Autodesk Inventor part; units mm, degrees
ref_plane "YZ Plane" through (0, 0, 0) normal (1, 0, 0) x (0, 1, 0)
ref_plane "XZ Plane" through (0, 0, 0) normal (0, 1, 0) x (-1, 0, 0)
ref_plane "XY Plane" through (0, 0, 0) normal (0, 0, 1) x (1, 0, 0)
sketch "Sketch1" plane through (0, 0, 0) normal (0, 0, 1) x (1, 0, 0)
  line L0 (0, 0) -> (30.25, 0) construction
  line L1 (0, 0) -> (-30.25, 0) construction
  line L2 (-30.25, 0) -> (-30.25, 40) construction
  line L3 (-30.25, 0) -> (-30.25, -40) construction
  circle A0 centre (-30.25, 40) radius 2.7
  circle A1 centre (-30.25, -40) radius 2.7
  circle A2 centre (30.25, 0) radius 2.7
  circle A3 centre (-30.25, 40) radius 12
  circle A4 centre (-30.25, -40) radius 12
  circle A5 centre (30.25, 0) radius 12
  line L4 (36.868172, -10.009985) -> (-23.631828, -50.009985)
  line L5 (-42.25, 40) -> (-42.25, -40)
  circle A6 centre (-34.25, 0) radius 2
  line L6 (-30.25, 0) -> (-34.25, 0) construction
  line L7 (-23.631828, 50.009985) -> (36.868172, 10.009985)
  line L8 (30.25, 0) -> (50.25, 0) construction
  circle A7 centre (50.25, 0) radius 10
  circle A8 centre (50.25, 0) radius 2
  line L9 (50.25746, 9.999997) -> (36.868172, 10.009985)
  line L10 (50.25746, -9.999997) -> (36.868172, -10.009985)
  circle A9 centre (10.25, 0) radius 2
  line L11 (50.25746, -9.999997) -> (60.257457, -9.992538)
  line L12 (60.257457, -9.992538) -> (60.242549, 9.992549)
  line L13 (60.242549, 9.992549) -> (50.25746, 9.999997)
  point P0 (-42.25, 0)
  point P1 (41.35, -4.559605)
  point P2 (41.35, 4.559605)
  point P3 (60.249997, 0.00746)
  dimension "d0" = 60.5
  dimension "d1" = 5.4
  dimension "d2" = 80
  dimension "d3" = 24
  dimension "d55" = 4
  dimension "d56" = 8
  dimension "d57" = 20
  dimension "d58" = 20
  dimension "d69" = 20
sketch "Sketch1 outline for Extrusion1" plane through (0, 0, 0) normal (0, 0, 1) x (1, 0, 0)
  arc A0 (-23.631828, 50.009985) -> (-42.25, 40) centre (-30.25, 40) ccw
  line L0 (-42.25, 40) -> (-42.25, -40)
  arc A1 (-42.25, -40) -> (-23.631828, -50.009985) centre (-30.25, -40) ccw
  line L1 (-23.631828, -50.009985) -> (36.868172, -10.009985)
  line L2 (36.868172, -10.009985) -> (60.257457, -9.992538)
  line L3 (60.257457, -9.992538) -> (60.242549, 9.992549)
  line L4 (60.242549, 9.992549) -> (36.868172, 10.009985)
  line L5 (36.868172, 10.009985) -> (-23.631828, 50.009985)
  circle A2 centre (-30.25, 40) radius 2.7
  circle A3 centre (10.25, 0) radius 2
  circle A4 centre (-34.25, 0) radius 2
  circle A5 centre (30.25, 0) radius 2.7
  circle A6 centre (-30.25, -40) radius 2.7
  circle A7 centre (50.25, 0) radius 2
extrude "Extrusion1" add sketch "Sketch1 outline for Extrusion1" against normal blind 10
fillet "Fillet1" radius 20 2 edges at (36.8682, 10.01, -5) (36.8682, -10.01, -5)
chamfer "Chamfer6" distance 2 angle 45 2 edges at (60.2425, 9.9925, -5) (60.2575, -9.9925, -5)
sketch "Sketch8" plane through (0, 0, 0) normal (0, 0, 1) x (1, 0, 0)
  line L0 (58.257457, -9.99403) -> (60.255965, -7.992538)
  line L1 (58.257457, -9.99403) -> (42.873828, -10.005505)
  arc A0 (42.873828, -10.005505) -> (31.85846, -13.322191) centre (42.888747, -30.0055) ccw
  line L2 (31.85846, -13.322191) -> (-23.631828, -50.009985)
  arc A1 (-42.25, -40) -> (-23.631828, -50.009985) centre (-30.25, -40) ccw
  line L3 (-42.25, -40) -> (-42.25, 40)
  arc A2 (-23.631828, 50.009985) -> (-42.25, 40) centre (-30.25, 40) ccw
  line L4 (-23.631828, 50.009985) -> (31.85846, 13.322191)
  arc A3 (31.85846, 13.322191) -> (42.873828, 10.005505) centre (42.888747, 30.0055) ccw
  line L5 (42.873828, 10.005505) -> (58.242549, 9.994041)
  line L6 (60.244041, 7.992549) -> (58.242549, 9.994041)
  line L7 (60.244041, 7.992549) -> (60.255965, -7.992538)
  circle A4 centre (30.25, 0) radius 2.7
  circle A5 centre (50.25, 0) radius 2
  circle A6 centre (-30.25, -40) radius 2.7
  circle A7 centre (-34.25, 0) radius 2
  circle A8 centre (10.25, 0) radius 2
  circle A9 centre (-30.25, 40) radius 2.7
  line L8 (-28.200407, -43.55) -> (-32.299593, -43.55)
  line L9 (-32.299593, -43.55) -> (-34.349187, -40)
  line L10 (-34.349187, -40) -> (-32.299593, -36.45)
  line L11 (-32.299593, -36.45) -> (-28.200407, -36.45)
  line L12 (-28.200407, -36.45) -> (-26.150813, -40)
  line L13 (-26.150813, -40) -> (-28.200407, -43.55)
  line L14 (-28.200407, 36.45) -> (-32.299593, 36.45)
  line L15 (-32.299593, 36.45) -> (-34.349187, 40)
  line L16 (-34.349187, 40) -> (-32.299593, 43.55)
  line L17 (-32.299593, 43.55) -> (-28.200407, 43.55)
  line L18 (-28.200407, 43.55) -> (-26.150813, 40)
  line L19 (-26.150813, 40) -> (-28.200407, 36.45)
  line L20 (32.299593, -3.55) -> (28.200407, -3.55)
  line L21 (28.200407, -3.55) -> (26.150813, 0)
  line L22 (26.150813, 0) -> (28.200407, 3.55)
  line L23 (28.200407, 3.55) -> (32.299593, 3.55)
  line L24 (32.299593, 3.55) -> (34.349187, 0)
  line L25 (34.349187, 0) -> (32.299593, -3.55)
  point P0 (0, 0)
  dimension "d83" = 7.1
  dimension "d84" = 7.1
  dimension "d85" = 7.1
extrude "Extrusion9" cut sketch "Sketch8" against normal blind 3 contours L8 L9 L10 L11 L12 L13 | L14 L15 L16 L17 L18 L19 | L20 L21 L22 L23 L24 L25
sketch "Sketch5" plane through (0, 0, 0) normal (0, 0, 1) x (1, 0, 0)
  arc A0 (-42.25, -40) -> (-23.631828, -50.009985) centre (-30.25, -40) ccw
  line L0 (-23.631828, -50.009985) -> (31.85846, -13.322191)
  arc A1 (42.873828, -10.005505) -> (31.85846, -13.322191) centre (42.888747, -30.0055) ccw
  line L1 (42.873828, -10.005505) -> (58.257457, -9.99403)
  arc A2 (31.85846, 13.322191) -> (42.873828, 10.005505) centre (42.888747, 30.0055) ccw
  line L2 (31.85846, 13.322191) -> (-23.631828, 50.009985)
  arc A3 (-23.631828, 50.009985) -> (-42.25, 40) centre (-30.25, 40) ccw
  line L3 (-42.25, 40) -> (-42.25, -40)
  circle A4 centre (-34.25, 0) radius 2
  circle A5 centre (50.25, 0) radius 2
  line L4 (-4.75, 10.2) -> (-4.75, 37.526132)
  line L5 (-4.75, 10.2) -> (25.25, 10.2)
  line L6 (25.25, 10.2) -> (25.25, 17.691421)
  line L7 (60.255965, -7.992538) -> (60.244041, 7.992549)
  line L8 (58.242549, 9.994041) -> (42.873828, 10.005505)
  line L9 (60.255965, -7.992538) -> (58.257457, -9.99403)
  line L10 (58.242549, 9.994041) -> (60.244041, 7.992549)
  dimension "d66" = 30
  dimension "d92" = 10.2
  dimension "d93" = 25
extrude "Extrusion6" add sketch "Sketch5" along normal blind 20 contours L2 L6 L5 L4
sketch "Sketch9" plane through (0, 0, 20) normal (0, 0, 1) x (1, 0, 0)
  circle A0 centre (10.25, 0) radius 2
  line L0 (25.25, 10.2) -> (25.25, 17.691421)
  line L1 (25.25, 17.691421) -> (-4.75, 37.526132)
  line L2 (-4.75, 37.526132) -> (-4.75, 10.2)
  line L3 (-4.75, 10.2) -> (25.25, 10.2)
  line L4 (10.25, 0) -> (10.25, 17.5) construction
  circle A1 centre (10.25, 17.5) radius 2.5
  point P0 (0, 0)
  dimension "d88" = 17.5
  dimension "d89" = 5
extrude "Extrusion10" cut sketch "Sketch9" against normal blind 5 contours A1
mirror "Mirror1" about plane through (0, 0, 0) normal (0, 1, 0) of "Extrusion10", "Extrusion6"
equation "\"d84\" = d83"
equation "\"d85\" = d83"
equation "\"b\" = 2"
properties part number "y axis something back_3DPrint"
Geometry: final body of the model. Coordinates: model frame, mm. A direction names the side the tool comes from. Round coordinates to 2 decimals unless told otherwise and drop trailing zeros. Loops run counter-clockwise (first coordinate to the right, second up) from the corner with the lowest first, then second, coordinate; pieces in that order, holes last. Notation, with made-up numbers: M 62,-15.5 L 89,-15.5 A27 ccw 89,9.5 Z; hole C -29,-7.5 d7. An arc over 180 degrees is marked long. Put each result on its own line as item: value. Start each with the question number.
(1) Set-up query: faces 1 (the face through (-4.75, -24, 10)), 2 (the face through (-33.34, 41.75, -1.48)), 3 (the face through (8.663, -1.217, -4.93)), 4 (the face through (7, 21, 20)), 5 (the face through (10, -10.2, 10)). Return all of +Z, -Z, +X, -X, +Y, -Y with unobstructed straight access to the full face (end or side cutting, diameter ignored); none if empty.
(2) Section query C-C (x = -30.25). Return loops of the section in (y, z).
(3) Section query B-B (z = 3.75). Return loops of the section in (x, y), then the cut area to 3 significant figures.
(4) Section query D-D (x = 10.25). Return loops of the section in (y, z).
(5) Section query A-A (x = 50.25). Return loops of the section in (y, z).
(6) Draft query along Y for faces 6 (the face through (25.25, 14, 10)), 7 (the face through (9.71, -19.94, 17.54)), 8 (the face through (37.2, 10.83, -5.07)). Return one class per face: +Y half, -Y half, draft (parallel to the pull), parting line (faces both ways), or undercut.
(7) Material intervals for line 1 along X through (y, z) = (-17.5, 17); line 2 along X through (y, z) = (-11.5, 1.25); line 3 along Z through (x, y) = (-17.5, -21), sorted ascending. Write a range as [from, to].
(8) Contact query for flat-ended pins moving along their axis: pin 1 Ø8 at (x, y) = (-18.5, -24) entering from +Z; pin 2 Ø16 at (y, z) = (-21.5, 13.5) entering from -X; pin 3 Ø8 at (x, z) = (11.5, -1) entering from +Y. Output: stop coordinate, or through.
Findings below:
1. face 1: +Z, -X, +Y, -Y
1. face 2: +Z
1. face 3: +Z, -Z
1. face 4: +Z, +X, -X, +Y, -Y
1. face 5: +Z, +X, -X
2. outline: M -52,-10 L -42.7,-10 L -42.7,-3 L -43.55,-3 L -43.55,0 L -52,0 Z; M -37.3,-10 L 37.3,-10 L 37.3,-3 L 36.45,-3 L 36.45,0 L -36.45,0 L -36.45,-3 L -37.3,-3 Z; M 42.7,-10 L 52,-10 L 52,0 L 43.55,0 L 43.55,-3 L 42.7,-3 Z
3. outline: M -4.75,-37.53 L 25.25,-17.69 L 25.25,-10.2 L -4.75,-10.2 Z; M -4.75,10.2 L 25.25,10.2 L 25.25,17.69 L -4.75,37.53 Z
3. area: 1,040 mm2
4. outline: M -27.61,-10 L -2,-10 L -2,0 L -10.2,0 L -10.2,20 L -15,20 L -15,15 L -20,15 L -20,20 L -27.61,20 Z; M 2,-10 L 27.61,-10 L 27.61,20 L 20,20 L 20,15 L 15,15 L 15,20 L 10.2,20 L 10.2,0 L 2,0 Z
5. outline: M -10,-10 L -2,-10 L -2,0 L -10,0 Z; M 2,-10 L 10,-10 L 10,0 L 2,0 Z
6. face 6: draft
6. face 7: undercut
6. face 8: +Y half
7. line 1: x = [-4.75, 7.75], [12.75, 25.25]
7. line 2: x = [-4.75, 25.25]
7. line 3: z = [-10, 0]
8. pin 1: stops at z = 0
8. pin 2: stops at x = -4.75
8. pin 3: stops at y = 29.43
